The model under review builds one solid part; all positions refer to its coordinate system, in mm. Face numbers are marked on the shaded views. A direction names the side the tool comes from. Coordinates: 2 decimals unless noted, no trailing zeros. Order: outer loops, then holes, each group sorted by start corner. A loop starts at its lowest first (then second) coordinate and runs counter-clockwise, first axis right, second up.
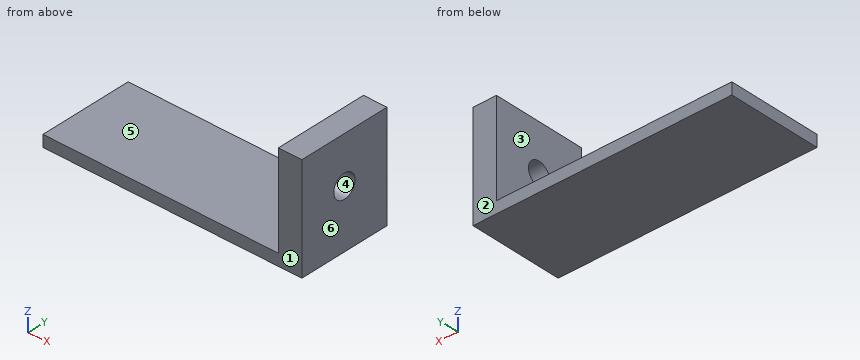
Solid Edge part; units mm, degrees
sketch "Sketch1" plane through (0, 0, 0) normal (0, 0, 1) x (1, 0, 0)
  line L0 (110, 40) -> (0, 40)
  line L1 (0, 40) -> (0, 0)
  line L2 (0, 0) -> (110, 0)
  line L3 (110, 0) -> (110, 40)
extrude "Protrusion1" add sketch "Sketch1" along normal blind 5
sketch "Sketch2" plane through (60, 20, 5) normal (0, 0, 1) x (1, 0, 0)
  line L0 (40, -20) -> (40, 20)
  line L1 (40, 20) -> (50, 20)
  line L2 (50, 20) -> (50, -20)
  line L3 (50, -20) -> (40, -20)
extrude "Extrusionsausprägung_2" add sketch "Sketch2" along normal blind 40
hole "Bohrung_1" at (110, 20, 25) direction (-1, 0, 0) diameter 10 end up to next
(1) Insertion check: pin 1 Ø3 at (x, y) = (69, 30) entering from +Z; pin 2 Ø16 at (y, z) = (20, 25) entering from -X. Each pin has a flat end and moves straight along its axis. Give the tip position at first contact, or say it passes through.
(2) Tool access review of the marked faces 5 and 6: name each direction out of +Z, -Z, +X, -X, +Y, -Y from which nothing blocks a thin tool from reaching the whole face with its end or side.
(3) The part is to be moulded in two halves that separate along Y. For the marked faces 1, 2, 3 and 4, say which applies: +Y half, -Y half, draft (parallel to the pull), parting line (faces both ways), or undercut.
(4) Consider section D-D (x = 84). Give the boundary of the cut face in (y, z), then the cut area to 3 significant figures.
(5) Consider section B-B (y = 20). Give the boundary of the cut face in (x, z).
(6) Consider section C-C (y = 29). Give the boundary of the cut face in (x, z).
(7) Consider section A-A (z = 25). Give the boundary of the cut face in (x, y), then the cut area to 3 significant figures.
(8) Wall thickness on line 1 (Z direction, x = 107, y = 20); line 2 (Y direction, x = 103, z = 25); line 3 (X direction, y = 15, z = 38.5): over which ranges is each line inside the solid? List them lowest first.
Findings:
1. pin 1: stops at z = 5
1. pin 2: stops at x = 100
2. face 5: +Z, -X, +Y, -Y
2. face 6: +Z, -Z, +X, +Y, -Y
3. face 1: -Y half
3. face 2: +Y half
3. face 3: draft
3. face 4: undercut
4. outline: (0, 0) - (40, 0) - (40, 5) - (0, 5) - close
4. area: 200 mm2
5. outline: (0, 0) - (110, 0) - (110, 20) - (100, 20) - (100, 5) - (0, 5) - close; (100, 30) - (110, 30) - (110, 45) - (100, 45) - close
6. outline: (0, 0) - (110, 0) - (110, 45) - (100, 45) - (100, 5) - (0, 5) - close
7. outline: (100, 0) - (110, 0) - (110, 15) - (100, 15) - close; (100, 25) - (110, 25) - (110, 40) - (100, 40) - close
7. area: 300 mm2
8. line 1: z = 0 to 20, 30 to 45
8. line 2: y = 0 to 15, 25 to 40
8. line 3: x = 100 to 110
